```python
from build123d import *

# Parameters (mm, degrees)
REVOLUTION_ANGLE     = -180
THICKNESS_T          = -1.3
POCKET_DEPTH         = 73.801
POCKET_DEPTH_BACK    = -73.801
SKETCH002_R          = 2
POCKET001_DEPTH      = 5
SKETCH003_W          = 150
SKETCH003_H          = 50
POCKET002_DEPTH      = 0.001
POCKET002_DEPTH_BACK = -48.044069


with BuildPart() as part:
    # Sketch → Revolution (revolve)
    with BuildSketch(Plane.XZ):
        Polygon((0, 0), (0, 52.6), (73.8, 38.6), (73.8, 0), align=None)
    revolve(axis=Axis((0, 0, 0), (0, 0, 1)), revolution_arc=REVOLUTION_ANGLE)

    # Thickness
    thickness_openings = [part.faces().sort_by_distance(p)[0] for p in [
        (0, 0, 22.979094),
    ]]
    offset(amount=THICKNESS_T, openings=thickness_openings)

    # Sketch001 → Pocket (cut, two sides)
    with BuildSketch(Plane.YZ) as pocket_sk:
        Polygon((0, 0), (-30, 60), (10, 60), (10, 0), align=None)
    extrude(amount=-POCKET_DEPTH, mode=Mode.SUBTRACT)
    extrude(pocket_sk.sketch, amount=-POCKET_DEPTH_BACK, mode=Mode.SUBTRACT)

    # Sketch002 → Pocket001 (cut)
    with BuildSketch(Plane.XY):
        with Locations((-50, -10)):
            Circle(SKETCH002_R)
        with Locations((50, -10)):
            Circle(SKETCH002_R)
    extrude(amount=POCKET001_DEPTH, mode=Mode.SUBTRACT)

    # Sketch003 → Pocket002 (cut, two sides)
    with BuildSketch(Plane.XY) as pocket002_sk:
        with Locations((0, -75)):
            Rectangle(SKETCH003_W, SKETCH003_H)
    extrude(amount=-POCKET002_DEPTH, mode=Mode.SUBTRACT)
    extrude(pocket002_sk.sketch, amount=-POCKET002_DEPTH_BACK, mode=Mode.SUBTRACT)


solid = part.part
```
Check sheet for the modelled part. Datum: model origin and axes. Units: mm. A direction names the side the tool comes from. Give positions to 0.01 mm unless a question says otherwise; leave off trailing zeros. Order: outer loops, then holes, each group sorted by start corner. A loop starts at its lowest first (then second) coordinate and runs counter-clockwise, first axis right, second up. Notation, with made-up numbers: M 22,-13.75 L 69,-13.75 A22 ccw 69,2.25 Z; hole C 60.25,76 d6. An arc over 180 degrees is marked long. Answer in a Markdown table with one row per item.
1) Cross-section at D-D, the plane x = -50. Count the separate pieces of the cut face and the enclosed holes in it, plus the area to 3 significant figures.
Filled sheet:
| item | result |
|---|---|
| separate pieces | 3 |
| enclosed holes | 0 |
| area | 98.0 mm2 |
2) Cross-section at A-A, the plane z = 4.5. Enter the section's corners in (x, y).
Filled sheet:
| item | result |
|---|---|
| outline | M -73.77,-2.25 A73.8 ccw -54.28,-50 L -52.5,-50 A72.5 cw -72.47,-2.25 Z; M 52.5,-50 L 54.28,-50 A73.8 ccw 73.77,-2.25 L 72.47,-2.25 A72.5 cw Z |
3) Access from +Z, -Z, +X, -X, +Y, -Y to the whole of each face (thin tool, end or side, straight path). Record for faces 4 (the conical face through (0.698, -38.191, 45.354)), 5 (the conical face through (0.685, -37.389, 44.183)).
Filled sheet:
| item | result |
|---|---|
| face 4 | +Z, -Y |
| face 5 | +Y |
4) Thickness scan on L1, parallel to X at y = -10, z = 0.95; L2, parallel to Y at x = -50, z = 1; L3, parallel to X at y = -44, z = 20.5. Record the ranges inside material, lowest first. Write a range as [from, to].
Filled sheet:
| item | result |
|---|---|
| L1 | x = [-73.12, -52], [-48, 48], [52, 73.12] |
| L2 | y = [-50, -12], [-8, -0.5] |
| L3 | x = [-59.25, -57.62], [57.62, 59.25] |
5) Cross-section at B-B, the plane y = -10. Enter the section's corners in (x, z), plus the area to 3 significant figures.
Filled sheet:
| item | result |
|---|---|
| outline | M -73.12,0 L -52,0 L -52,1.3 L -71.81,1.3 L -71.81,20 L -73.12,20 Z; M -48,0 L 48,0 L 48,1.3 L -48,1.3 Z; M 52,0 L 73.12,0 L 73.12,20 L 71.81,20 L 71.81,1.3 L 52,1.3 Z |
| area | 229 mm2 |
6) Release check for a two-part mould opening along Y. For faces 1 (the flat face through (-1, -25, 0)), 2 (the cylindrical face through (66.463, -32.079, 19.03)), 3 (the cylindrical face through (51.908, -9.399, 0.641)) record: +Y half, -Y half, draft (parallel to the pull), parting line (faces both ways), or undercut.
Filled sheet:
| item | result |
|---|---|
| face 1 | draft |
| face 2 | -Y half |
| face 3 | undercut |
7) Cross-section at C-C, the plane z = 16. Enter the section's corners in (x, y), plus the area to 3 significant figures.
Filled sheet:
| item | result |
|---|---|
| outline | M -73.37,-8 A73.8 ccw -54.28,-50 L -52.5,-50 A72.5 cw -72.06,-8 Z; M 52.5,-50 L 54.28,-50 A73.8 ccw 73.37,-8 L 72.06,-8 A72.5 cw Z |
| area | 122 mm2 |
8) Gauge pin test, flat ends, axial feed: P1, Ø1.5, axis at x = -34, y = -6, coming from the +Z side; P2, Ø5, axis at y = -37.5, z = 17.5, coming from the +X side; P3, Ø10, axis at y = -14, z = 23, coming from the +X side; P4, Ø2.5, axis at x = -50, y = -10, coming from the -Z side. Record the tip position at first contact, or that the pin passes through.
Filled sheet:
| item | result |
|---|---|
| P1 | stops at z = 1.3 |
| P2 | stops at x = 64.97 |
| P3 | stops at x = 73.12 |
| P4 | passes through |
